The model under review builds one solid part; all positions refer to its coordinate system, in mm. A direction names the side the tool comes from. Coordinates: 2 decimals unless noted, no trailing zeros. Order: outer loops, then holes, each group sorted by start corner. A loop starts at its lowest first (then second) coordinate and runs counter-clockwise, first axis right, second up. Notation, with made-up numbers: (73, 39) -> (85, 39) arc R22 cw to (85, 77) -> close; hole circle Ø5 at (33.25, 54). An arc over 180 degrees is marked (long way). Use one line per item in the form item = value.
from build123d import *

# Parameters (mm, degrees)
F0_R     = 3.175
F1_DEPTH = 25.4


with BuildPart() as f1:
    # F0 (on Front) → F1 (new body)
    with BuildSketch(Plane.XZ):
        with BuildLine():
            ThreePointArc((-9.5239774035, 114.4395686855), (-0.0697862158, 104.7752556526), (9.525, 114.3))
            ThreePointArc((9.525, 114.3), (9.5222292979, 114.5297263555), (9.5139188035, 114.759319062))
            ThreePointArc((9.5139188035, 114.759319062), (-0.1599542737, 123.8236568413), (-9.5239774035, 114.4395686855))
        make_face()
        with Locations((0, 114.3)):
            Circle(F0_R, mode=Mode.SUBTRACT)
        with BuildLine():
            ThreePointArc((52.3875, 0), (50.1616327839, 5.5119104847), (44.7324052746, 7.9324746146))
            ThreePointArc((44.7324052746, 7.9324746146), (36.5125, 0), (44.7324052746, -7.9324746146))
            ThreePointArc((44.7324052746, -7.9324746146), (50.1616327839, -5.5119104847), (52.3875, 0))
        make_face()
        with Locations((44.45, 0)):
            Circle(F0_R, mode=Mode.SUBTRACT)
        with BuildLine():
            ThreePointArc((15.875, 63.5), (15.651593952, 66.1539087707), (14.9876637149, 68.7331215703))
            ThreePointArc((14.9876637149, 68.7331215703), (-0.0901164538, 79.3747442192), (-15.0461097884, 68.5626282933))
            ThreePointArc((-15.0461097884, 68.5626282933), (-15.7758551867, 65.2714452088), (-15.7942028036, 61.9003804205))
            ThreePointArc((-15.7942028036, 61.9003804205), (-1.3691563451, 47.6841523812), (15.2843424201, 59.2099531722))
            ThreePointArc((15.2843424201, 59.2099531722), (15.7266423772, 61.3347414611), (15.875, 63.5))
        make_face()
        with Locations((0, 63.5)):
            Circle(F0_R, mode=Mode.SUBTRACT)
        with BuildLine():
            ThreePointArc((15.2843424201, 59.2099531722), (-1.3691563451, 47.6841523812), (-15.7942028036, 61.9003804205))
            Line((-15.7942028036, 61.9003804205), (-9.525, 0))
            ThreePointArc((-9.525, 0), (-6.7351920908, 6.7351920908), (0, 9.525))
            ThreePointArc((0, 9.525), (0.3388863295, 9.5189695375), (0.6773435479, 9.500885786))
            ThreePointArc((0.6773435479, 9.500885786), (6.9705567315, 6.4912990883), (9.525, 0))
            ThreePointArc((9.525, 0), (6.9705567315, -6.4912990883), (0.6773435479, -9.500885786))
            Line((0.6773435479, -9.500885786), (44.7324052746, -7.9324746146))
            ThreePointArc((44.7324052746, -7.9324746146), (36.5125, 0), (44.7324052746, 7.9324746146))
            Line((44.7324052746, 7.9324746146), (18.8638606461, 8.8534247346))
            ThreePointArc((18.8638606461, 8.8534247346), (13.1651151548, 11.5615969219), (11.2338630667, 17.5682733858))
            Line((11.2338630667, 17.5682733858), (15.2843424201, 59.2099531722))
        make_face()
        with BuildLine():
            ThreePointArc((0, 9.525), (-6.7351920908, 6.7351920908), (-9.525, 0))
            ThreePointArc((-9.525, 0), (-6.7351920908, -6.7351920908), (0, -9.525))
            Line((0, -9.525), (0.6773435479, -9.500885786))
            ThreePointArc((0.6773435479, -9.500885786), (6.9705567315, -6.4912990883), (9.525, 0))
            ThreePointArc((9.525, 0), (6.9705567315, 6.4912990883), (0.6773435479, 9.500885786))
            Line((0.6773435479, 9.500885786), (0, 9.525))
        make_face()
        with BuildLine():
            Line((0.6773435479, -9.500885786), (0, -9.525))
            ThreePointArc((0, -9.525), (0.3388863295, -9.5189695375), (0.6773435479, -9.500885786))
        make_face()
        with BuildLine():
            ThreePointArc((0.6773435479, 9.500885786), (0.3388863295, 9.5189695375), (0, 9.525))
            Line((0, 9.525), (0.6773435479, 9.500885786))
        make_face()
        with BuildLine():
            ThreePointArc((9.5139188035, 114.759319062), (9.5222292979, 114.5297263555), (9.525, 114.3))
            ThreePointArc((9.525, 114.3), (-0.0697862158, 104.7752556526), (-9.5239774035, 114.4395686855))
            Line((-9.5239774035, 114.4395686855), (-15.0461097884, 68.5626282933))
            ThreePointArc((-15.0461097884, 68.5626282933), (-0.0901164538, 79.3747442192), (14.9876637149, 68.7331215703))
            Line((14.9876637149, 68.7331215703), (9.5139188035, 114.759319062))
        make_face()
        with Locations((-6.0980641283, 100.0252)):
            Circle(F0_R, mode=Mode.SUBTRACT)
    extrude(amount=F1_DEPTH)


solid = f1.part
Item 1: We need section C-C (x = 8). Write out the cut boundary in (y, z).
Results found:
outline = (-25.4, -9.24) -> (0, -9.24) -> (0, 119.47) -> (-25.4, 119.47) -> close
Item 2: We need section D-D (z = 36). Write out the cut boundary in (x, y).
Results found:
outline = (-13.17, -25.4) -> (13.03, -25.4) -> (13.03, 0) -> (-13.17, 0) -> close
Item 3: Clearance check with flat-ended pins moving along their axes: pin 1 (5.5 mm diameter, centred on x = 0, z = 63.5, fed in from +Y); pin 2 (6 mm diameter, centred on y = -20.5, z = 37.5, fed in from +X); pin 3 (8 mm diameter, centred on y = -7, z = 91, fed in from +X); pin 4 (1 mm diameter, centred on y = -13.5, z = 45.5, fed in from -X). State where each tip first meets the part, or that it passes through.
Results found:
pin_1 = through
pin_2 = 13.46
pin_3 = 12.82
pin_4 = -14.18
Item 4: We need section A-A (z = 113). Write out the cut boundary in (x, y).
Results found:
outline = (-9.7, -25.4) -> (-2.9, -25.4) -> (-2.9, 0) -> (-9.7, 0) -> close; (2.9, -25.4) -> (9.72, -25.4) -> (9.72, 0) -> (2.9, 0) -> close
Item 5: To check wall thickness, follow L1, parallel to Z at x = -2.5, y = -18; L2, parallel to X at y = -14.25, z = 117; L3, parallel to Z at x = 21, y = -13. State the ranges of each line that lie inside material, in increasing order. Write a range as from..to.
Results found:
L1 = -9.19..61.54, 65.46..112.34, 116.26..123.49
L2 = -9.13..-1.67, 1.67..9.13
L3 = -8.78..8.78
Item 6: Draft analysis for pull direction X (two halves, no side actions). For faces 1 (the face through (-0.69, -12.52, 111.2)), 2 (the face through (3, -25.4, 43)), 3 (the face through (-12.246, -12.522, 91.822)), state which applies: released by +X, released by -X, zero draft, split by the parting line, or undercut.
Results found:
face_1 = undercut
face_2 = zero draft
face_3 = released by -X
Item 7: We need section B-B (y = -23). State how many separate pieces and enclosed holes the cut face has, plus the area to 3 significant figures.
Results found:
separate_pieces = 1
enclosed_holes = 4
area = 3,780 mm²
Item 8: Tool access review of faces 4 (the face through (41.28, -12.52, 0.14)), 5 (the face through (13.23, -12.52, 38.1)): name each direction out of +Z, -Z, +X, -X, +Y, -Y from which nothing blocks a thin tool from reaching the whole face with its end or side.
Results found:
face_4 = +Y, -Y
face_5 = +X, +Y, -Y
